The figure shows three views and two pictorial views of one solid part (mm, origin at its lowest corner). Answer the questions. A direction names the side the tool comes from. Coordinates: 2 decimals unless noted, no trailing zeros. Loops run counter-clockwise (first coordinate to the right, second up) from the corner with the lowest first, then second, coordinate; pieces in that order, holes last. Notation, with made-up numbers: (86.25, 39.25) - (107.25, 39.25) arc R16 cw to (107.25, 43.25) - close; hole circle Ø1 at (-36, 11.25). An arc over 180 degrees is marked (long way). One line per question, with ' | ' between items.
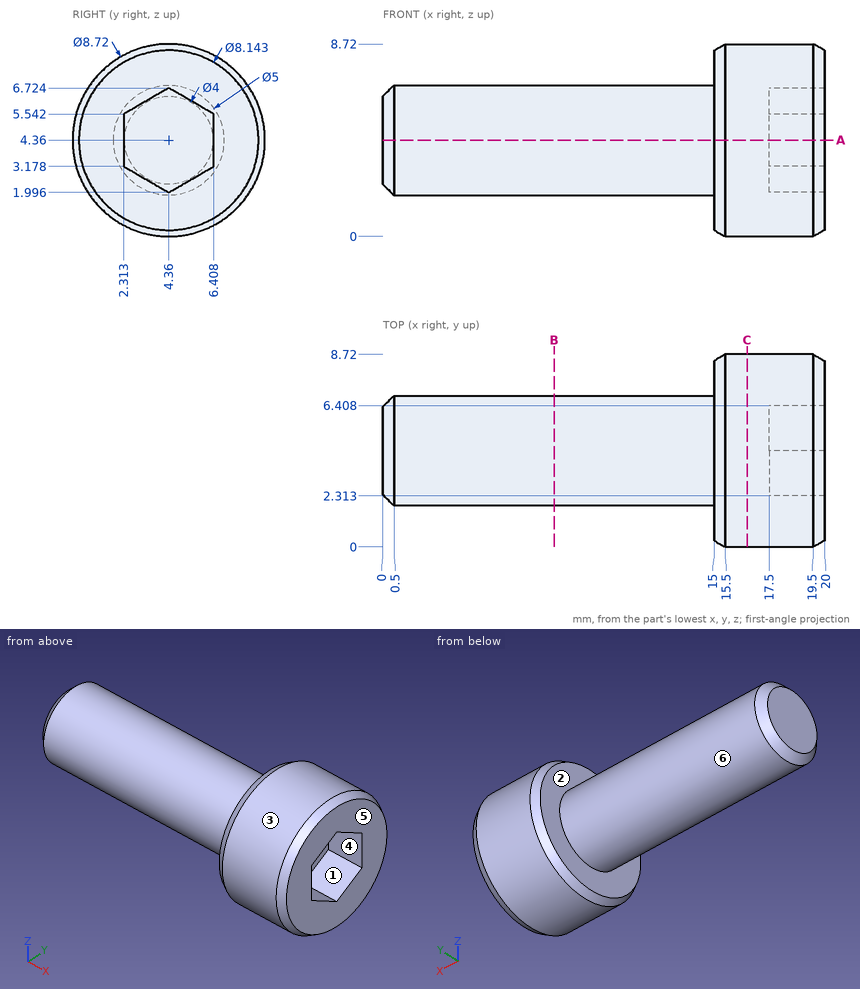
Item 1: Which of the six approach directions +Z, -Z, +X, -X, +Y, -Y give full straight-line access (tool end or side, diameter ignored) to the marked faces 5 and 6?
Taken from the geometry:
face 5: +Z, -Z, +X, +Y, -Y | face 6: -X
Item 2: Each of these flat-tipped pins is pushed along its axis until it touches: pin 1 Ø3 at (x, z) = (14, 5.5) entering from +Y (1 decimal); pin 2 Ø1.9 at (x, z) = (18.5, 5) entering from -Y; pin 3 Ø1 at (x, y) = (2.5, 3.5) entering from -Z; pin 4 Ø1 at (x, z) = (8, 4) entering from +Y. Where does it stop, or does it pass through?
Taken from the geometry:
pin 1: stops at y = 8.6 | pin 2: stops at y = 0 | pin 3: stops at z = 1.89 | pin 4: stops at y = 6.86
Item 3: Find section A-A, the plane z = 4.36. Write down the section's boundary in (x, y).
Taken from the geometry:
outline: (0, 2.36) - (0.5, 1.86) - (15, 1.86) - (15, 0.29) - (15.5, 0) - (19.5, 0) - (20, 0.29) - (20, 2.31) - (17.5, 2.31) - (17.5, 6.41) - (20, 6.41) - (20, 8.43) - (19.5, 8.72) - (15.5, 8.72) - (15, 8.43) - (15, 6.86) - (0.5, 6.86) - (0, 6.36) - close
Item 4: The mould has two halves that part along Y. Classify the marked faces 1, 2, 3 and 4: pulls with the +Y half, pulls with the -Y half, needs draft (parallel to the pull), parting line crosses it, or undercut.
Taken from the geometry:
face 1: undercut | face 2: needs draft | face 3: parting line crosses it | face 4: undercut
Item 5: Find the intervals of material crossed by line 1 (Y direction, x = 18.5, z = 4.5); line 2 (X direction, y = 5.25, z = 2.25); line 3 (X direction, y = 3.25, z = 7.75), in increasing order. Write a range as [from, to].
Taken from the geometry:
line 1: y = [0, 2.31], [6.41, 8.72] | line 2: x = [0.29, 20] | line 3: x = [15, 20]
Item 6: Find section C-C, the plane x = 16.5. Write down the section's boundary in (y, z).
Taken from the geometry:
outline: circle Ø8.72 at (4.36, 4.36)
Item 7: Find section B-B, the plane x = 7.75. Write down the section's boundary in (y, z).
Taken from the geometry:
outline: circle Ø5 at (4.36, 4.36)
